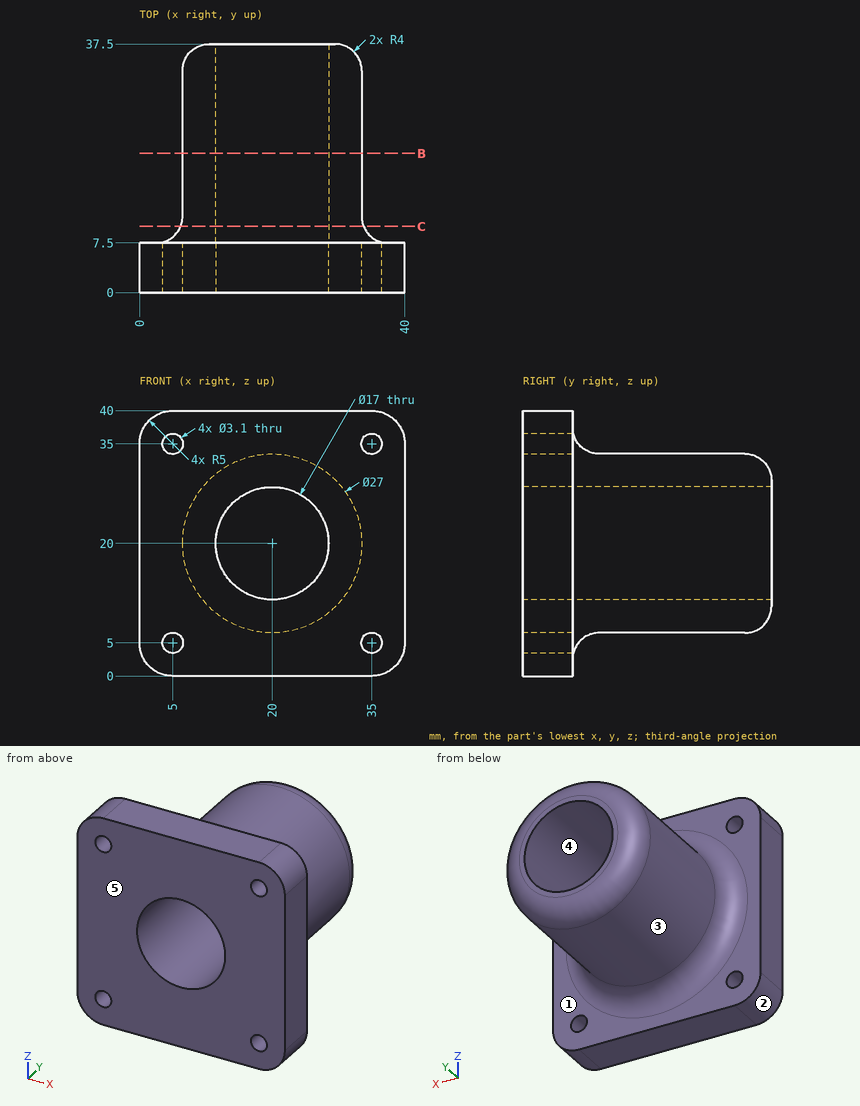
Study the drawing (mm; zero at the part's minimum x, y, z) and answer. A direction names the side the tool comes from. Coordinates: 2 decimals unless noted, no trailing zeros. Loops run counter-clockwise (first coordinate to the right, second up) from the corner with the lowest first, then second, coordinate; pieces in that order, holes last. Notation, with made-up numbers: M -34.75,-28 L 3.25,-28 A27 cw 3.25,7 Z; hole C -17.75,61.5 d11. An arc over 180 degrees is marked long. Answer in a Markdown table with one row per item. Add a question column.
1. Find section C-C, the plane y = 10. Write down the section's boundary in (x, z).
2. Find section B-B, the plane y = 21. Write down the section's boundary in (x, z).
3. The mould has two halves that part along X. Classify the marked faces 3, 4 and 5: pulls with the +X half, pulls with the -X half, needs draft (parallel to the pull), parting line crosses it, or undercut.
4. Flat-ended cylindrical pins translate along their axes: P1, Ø3, axis at x = 6.5, y = 26, coming from the +Z side; P2, Ø1.5, axis at y = 13.5, z = 24, coming from the -X side; P3, Ø3, axis at x = 35, z = 35, coming from the -Y side; P4, Ø5, axis at x = 5, z = 5, coming from the +Y side. Find the tip coordinate at first contact, or state that the pin passes through.
5. Consider L1, parallel to Z at x = 35, y = 2; L2, parallel to Z at x = 20, y = 14. Determine where each line is inside the solid, lowest interval first.
6. A tool of negligible diameter and unlimited length cuts with its end or side. For the marked faces 1 and 2, from which of +Z, -Z, +X, -X, +Y, -Y can it reach the whole face along a straight path? Write none if from no direction.
Reported:
| question | item | result |
|---|---|---|
| 1 | outline | C 20,20 d27.58; hole C 20,20 d17 |
| 2 | outline | C 20,20 d27; hole C 20,20 d17 |
| 3 | face 3 | parting line crosses it |
| 3 | face 4 | undercut |
| 3 | face 5 | needs draft |
| 4 | P1 | stops at z = 26.18 |
| 4 | P2 | stops at x = 6.9 |
| 4 | P3 | passes through |
| 4 | P4 | stops at y = 7.5 |
| 5 | L1 | z = 0 to 3.45, 6.55 to 33.45, 36.55 to 40 |
| 5 | L2 | z = 6.5 to 11.5, 28.5 to 33.5 |
| 6 | face 1 | +Y |
| 6 | face 2 | -Z, -X, +Y, -Y |
